from build123d import *

# Parameters (mm, degrees)
F0_R     = 3.45
F1_DEPTH = 6
F0_W     = 10
F0_H     = 41.4
F2_DEPTH = 11.8
F3_DEPTH = 34.5
F0_W_2   = 15
F0_H_2   = 3.8
F4_DEPTH = 35.15
F0_H_3   = 10.8
F0_R_2   = 2.25
F5_DEPTH = 21.667
F6_DEPTH = 22.1
F0_R_3   = 1.75
F7_DEPTH = 2.6
F8_DEPTH = 11.5


with BuildPart() as f1:
    # F0 (on Front) → F1 (new body)
    with BuildSketch(Plane.XZ):
        Polygon((15.5, 21), (-29.5, 21), (-29.5, 20.7), (-29.5, -20.7), (-29.5, -21), (15.5, -21), align=None)
        Polygon((-15.15, -13.607328), (-15.15, -9.392672), (-11.5, -7.285343), (-7.85, -9.392672), (-7.85, -13.607328), (-11.5, -15.714657), align=None, mode=Mode.SUBTRACT)
        Polygon((11.5, -15.714657), (7.85, -13.607328), (7.85, -9.392672), (11.5, -7.285343), (15.15, -9.392672), (15.15, -13.607328), align=None, mode=Mode.SUBTRACT)
        with Locations((-12, 1.5)):
            Circle(F0_R, mode=Mode.SUBTRACT)
        Polygon((-11.5, 15.714657), (-7.85, 13.607328), (-7.85, 9.392672), (-11.5, 7.285343), (-15.15, 9.392672), (-15.15, 13.607328), align=None, mode=Mode.SUBTRACT)
        with Locations((12, 1.5)):
            Circle(F0_R, mode=Mode.SUBTRACT)
        Polygon((7.85, 9.392672), (7.85, 13.607328), (11.5, 15.714657), (15.15, 13.607328), (15.15, 9.392672), (11.5, 7.285343), align=None, mode=Mode.SUBTRACT)
    extrude(amount=F1_DEPTH)

    # F0 (on Front) → F2 (join)
    with BuildSketch(Plane.XZ):
        with Locations((-34.5, 0)):
            Rectangle(F0_W, F0_H)
        Polygon((15.5, 21.35), (15.5, 21), (15.5, -21), (15.5, -21.35), (30.5, -21.35), (30.5, 21.35), align=None)
    extrude(amount=F2_DEPTH)

    # F0 (on Front) → F3 (join)
    with BuildSketch(Plane.XZ):
        Polygon((-29.5, 24.5), (-39.5, 24.5), (-39.5, 20.7), (-29.5, 20.7), (-29.5, 21), align=None)
        Polygon((-29.5, -20.7), (-39.5, -20.7), (-39.5, -24.5), (-29.5, -24.5), (-29.5, -21), align=None)
    extrude(amount=F3_DEPTH)

    # F0 (on Front) → F4 (join)
    with BuildSketch(Plane.XZ):
        with Locations((23, -23.25)):
            Rectangle(F0_W_2, F0_H_2)
        with Locations((23, 23.25)):
            Rectangle(F0_W_2, F0_H_2)
    extrude(amount=F4_DEPTH)

    # F0 (on Front) → F5 (join)
    with BuildSketch(Plane.XZ):
        with Locations((-34.5, -29.9)):
            Rectangle(F0_W, F0_H_3)
        Polygon((-34.5, -25.185343), (-30.85, -27.292672), (-30.85, -31.507328), (-34.5, -33.614657), (-38.15, -31.507328), (-38.15, -27.292672), align=None, mode=Mode.SUBTRACT)
        Polygon((-30.85, -31.507328), (-30.85, -27.292672), (-34.5, -25.185343), (-38.15, -27.292672), (-38.15, -31.507328), (-34.5, -33.614657), align=None)
        with Locations((-34.5, -29.4)):
            Circle(F0_R_2, mode=Mode.SUBTRACT)
        with Locations((-34.5, 29.9)):
            Rectangle(F0_W, F0_H_3)
        Polygon((-34.5, 33.614657), (-30.85, 31.507328), (-30.85, 27.292672), (-34.5, 25.185343), (-38.15, 27.292672), (-38.15, 31.507328), align=None, mode=Mode.SUBTRACT)
        Polygon((-30.85, 27.292672), (-30.85, 31.507328), (-34.5, 33.614657), (-38.15, 31.507328), (-38.15, 27.292672), (-34.5, 25.185343), align=None)
        with Locations((-34.5, 29.4)):
            Circle(F0_R_2, mode=Mode.SUBTRACT)
    extrude(amount=F5_DEPTH)

    # F0 (on Front) → F6 (join)
    with BuildSketch(Plane.XZ):
        with Locations((23, -30.55)):
            Rectangle(F0_W_2, F0_H_3)
        Polygon((26.65, -27.942672), (26.65, -32.157328), (23, -34.264657), (19.35, -32.157328), (19.35, -27.942672), (23, -25.835343), align=None, mode=Mode.SUBTRACT)
        Polygon((23, -34.264657), (26.65, -32.157328), (26.65, -27.942672), (23, -25.835343), (19.35, -27.942672), (19.35, -32.157328), align=None)
        with Locations((23, -30.05)):
            Circle(F0_R_2, mode=Mode.SUBTRACT)
        with Locations((23, 30.55)):
            Rectangle(F0_W_2, F0_H_3)
        Polygon((23, 34.264657), (26.65, 32.157328), (26.65, 27.942672), (23, 25.835343), (19.35, 27.942672), (19.35, 32.157328), align=None, mode=Mode.SUBTRACT)
        Polygon((26.65, 27.942672), (26.65, 32.157328), (23, 34.264657), (19.35, 32.157328), (19.35, 27.942672), (23, 25.835343), align=None)
        with Locations((23, 30.05)):
            Circle(F0_R_2, mode=Mode.SUBTRACT)
    extrude(amount=F6_DEPTH)

    # F0 (on Front) → F7 (join)
    with BuildSketch(Plane.XZ):
        Polygon((-7.85, 9.392672), (-7.85, 13.607328), (-11.5, 15.714657), (-15.15, 13.607328), (-15.15, 9.392672), (-11.5, 7.285343), align=None)
        with Locations((-11.5, 11.5)):
            Circle(F0_R_2, mode=Mode.SUBTRACT)
        Polygon((11.5, 15.714657), (7.85, 13.607328), (7.85, 9.392672), (11.5, 7.285343), (15.15, 9.392672), (15.15, 13.607328), align=None)
        with Locations((11.5, 11.5)):
            Circle(F0_R_2, mode=Mode.SUBTRACT)
        Polygon((7.85, -9.392672), (7.85, -13.607328), (11.5, -15.714657), (15.15, -13.607328), (15.15, -9.392672), (11.5, -7.285343), align=None)
        with Locations((11.5, -11.5)):
            Circle(F0_R_2, mode=Mode.SUBTRACT)
        Polygon((-11.5, -7.285343), (-15.15, -9.392672), (-15.15, -13.607328), (-11.5, -15.714657), (-7.85, -13.607328), (-7.85, -9.392672), align=None)
        with Locations((-11.5, -11.5)):
            Circle(F0_R_2, mode=Mode.SUBTRACT)
        with Locations((-12, 1.5)):
            Circle(F0_R)
        with Locations((-12, 1.5)):
            Circle(F0_R_3, mode=Mode.SUBTRACT)
        with Locations((12, 1.5)):
            Circle(F0_R)
        with Locations((12, 1.5)):
            Circle(F0_R_3, mode=Mode.SUBTRACT)
    extrude(amount=F7_DEPTH)

    # F0 (on Front) → F8 (cut)
    with BuildSketch(Plane.XZ):
        Polygon((23, -34.264657), (26.65, -32.157328), (26.65, -27.942672), (23, -25.835343), (19.35, -27.942672), (19.35, -32.157328), align=None)
        with Locations((23, -30.05)):
            Circle(F0_R_2, mode=Mode.SUBTRACT)
        Polygon((26.65, 27.942672), (26.65, 32.157328), (23, 34.264657), (19.35, 32.157328), (19.35, 27.942672), (23, 25.835343), align=None)
        with Locations((23, 30.05)):
            Circle(F0_R_2, mode=Mode.SUBTRACT)
        Polygon((-30.85, 27.292672), (-30.85, 31.507328), (-34.5, 33.614657), (-38.15, 31.507328), (-38.15, 27.292672), (-34.5, 25.185343), align=None)
        with Locations((-34.5, 29.4)):
            Circle(F0_R_2, mode=Mode.SUBTRACT)
        Polygon((-30.85, -31.507328), (-30.85, -27.292672), (-34.5, -25.185343), (-38.15, -27.292672), (-38.15, -31.507328), (-34.5, -33.614657), align=None)
        with Locations((-34.5, -29.4)):
            Circle(F0_R_2, mode=Mode.SUBTRACT)
    extrude(amount=F8_DEPTH, mode=Mode.SUBTRACT)


solid = f1.part
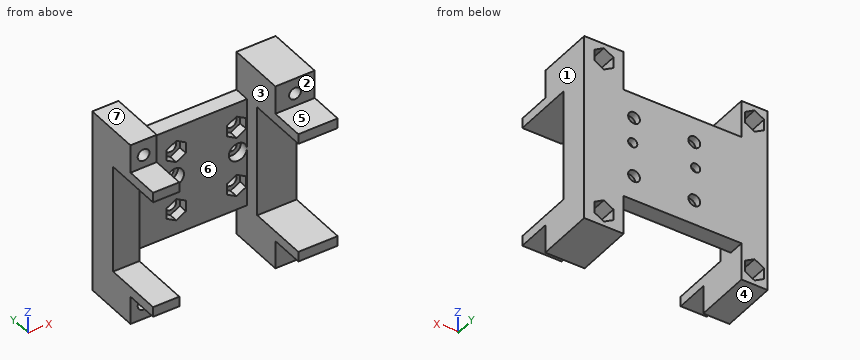
Can you work these out from the model? Positions are in its coordinate system, mm. Face numbers are marked on the shaded views. A direction names the side the tool comes from. Coordinates: 2 decimals unless noted, no trailing zeros. Write each loop counter-clockwise with the first axis right and the second up, starting at its lowest first coordinate (ties: lowest second). Pieces come first, ordered by that corner, then holes. Notation, with made-up numbers: (-5.5, 44) -> (22.5, 44) arc R30 ccw to (22.5, 83) -> close; hole circle Ø7 at (-0.75, 80.25). An arc over 180 degrees is marked (long way). Write each question's results on one line, items separated by ' | '. Start each with the question number.
Q1. Imagine slicing it at D-D (z = 1.5). Write out the boundary of the cut face in (x, y), then the cut area to 3 significant figures.
Q2. Imagine slicing it at C-C (y = -9.5). State how many separate pieces and enclosed holes the cut face has, then the cut area to 3 significant figures.
Q3. Imagine slicing it at B-B (z = 11.5). Write out the boundary of the cut face in (x, y).
Q4. We'd pull the mould along X, two halves only. Please class the marked faces 1, 2 and 3: +X half, -X half, draft (parallel to the pull), parting line (faces both ways), or undercut.
Q5. On a 3-axis mill with a long thin cutter (end or side, diameter ignored), from which of +Z, -Z, +X, -X, +Y, -Y can I reach the whole of each face in a straight line? I mean the marked faces 4, 5, 6 and 7. Say none if no direction works.
Q6. If I drill on probe 1 along Z at (x, y) = (-34.5, -14.25); probe 2 along X at (y, z) = (-5.5, -25); probe 3 along Z at (x, y) = (12, -4.1), over which ranges is the centre line in solid material (lowest first)?
Q7. Imagine slicing it at A-A (y = -19). Write out the boundary of the cut face in (x, z), then the cut area to 3 significant figures.
Q8. I'm going to push flat-ended pins straight in: pin 1 (5 mm diameter, centred on x = -35, y = -12.5, fed in from -Z); pin 2 (12 mm diameter, centred on x = 20, z = -31.5, fed in from -Y); pin 3 (10 mm diameter, centred on x = -28.5, y = -31.5, fed in from +Z). Where does each tip first touch, or does it pass through?
Taken from the geometry:
1) outline: (-39.5, -11.8) -> (-29.5, -11.8) -> (-29.5, -6) -> (-15.45, -6) -> (-15.45, -2.6) -> (-13.75, -2.6) -> (-13.75, 0) -> (-39.5, 0) -> close; (-10.25, -2.6) -> (-8.55, -2.6) -> (-8.55, -6) -> (8.55, -6) -> (8.55, -2.6) -> (10.25, -2.6) -> (10.25, 0) -> (-10.25, 0) -> close; (13.75, -2.6) -> (15.45, -2.6) -> (15.45, -6) -> (15.5, -6) -> (15.5, -11.8) -> (30.5, -11.8) -> (30.5, 0) -> (13.75, 0) -> close | area: 500 mm^2
2) separate pieces: 2 | enclosed holes: 4 | area: 1,600 mm^2
3) outline: (-39.5, -11.8) -> (-29.5, -11.8) -> (-29.5, -6) -> (-15.15, -6) -> (-15.15, -2.6) -> (-13.75, -2.6) -> (-13.75, 0) -> (-39.5, 0) -> close; (-9.25, -2.6) -> (-7.85, -2.6) -> (-7.85, -6) -> (7.85, -6) -> (7.85, -2.6) -> (9.25, -2.6) -> (9.25, 0) -> (-9.25, 0) -> close; (13.75, -2.6) -> (15.15, -2.6) -> (15.15, -6) -> (15.5, -6) -> (15.5, -11.8) -> (30.5, -11.8) -> (30.5, 0) -> (13.75, 0) -> close
4) face 1: +X half | face 2: draft | face 3: undercut
5) face 4: -Z, -X, +Y, -Y | face 5: +Z, +X, -X, -Y | face 6: +Z, -Z, -Y | face 7: +Z, -X, +Y, -Y
6) probe 1: z = -35.3 to -31.65, -27.15 to -20.7, 20.7 to 27.15, 31.65 to 35.3 | probe 2: x = -39.5 to -29.5, 15.5 to 30.5 | probe 3: z = -21 to -15.43, -7.57 to -1.95, 4.95 to 7.57, 15.43 to 21
7) outline: (-39.5, -35.3) -> (-29.5, -35.3) -> (-29.5, -20.7) -> (-39.5, -20.7) -> close; (-39.5, 20.7) -> (-29.5, 20.7) -> (-29.5, 35.3) -> (-39.5, 35.3) -> close; (15.5, -35.95) -> (30.5, -35.95) -> (30.5, -21.35) -> (15.5, -21.35) -> close; (15.5, 21.35) -> (30.5, 21.35) -> (30.5, 35.95) -> (15.5, 35.95) -> close; hole circle Ø4.5 at (-34.5, -29.4); hole circle Ø4.5 at (-34.5, 29.4); hole circle Ø4.5 at (23, -30.05); hole circle Ø4.5 at (23, 30.05) | area: 666 mm^2
8) pin 1: stops at z = -35.3 | pin 2: stops at y = -22.1 | pin 3: stops at z = 24.5
